Read the model definition and answer for the solid it produces. Units are mm, in the model's axes. Round coordinates to 2 decimals unless told otherwise and drop trailing zeros. Write each loop counter-clockwise with the first axis right and the second up, starting at its lowest first coordinate (ties: lowest second). Pieces come first, ordered by that corner, then holes.
from build123d import *

# Parameters (mm, degrees)
F0_R     = 1.5
F1_DEPTH = 3


with BuildPart() as f1:
    # F0 (on Top) → F1 (new body)
    with BuildSketch(Plane.XY):
        with BuildLine():
            Line((14, 6), (0, 6))
            ThreePointArc((0, 6), (-4.834596, 3.553404), (-5.726424, -1.791107))
            Line((-5.726424, -1.791107), (1.273576, -24.171107))
            ThreePointArc((1.273576, -24.171107), (7, -28.38), (12.726424, -24.171107))
            Line((12.726424, -24.171107), (19.726424, -1.791107))
            ThreePointArc((19.726424, -1.791107), (18.834596, 3.553404), (14, 6))
        make_face()
        with Locations((7, -22.38)):
            Circle(F0_R, mode=Mode.SUBTRACT)
        with Locations((7, -15)):
            Circle(F0_R, mode=Mode.SUBTRACT)
        with Locations((7, -7.62)):
            Circle(F0_R, mode=Mode.SUBTRACT)
        Circle(F0_R, mode=Mode.SUBTRACT)
        with Locations((14, 0)):
            Circle(F0_R, mode=Mode.SUBTRACT)
    extrude(amount=F1_DEPTH)


solid = f1.part
Q1. Section B-B (x = 7) is taken. Determine the outline of the cut face in (y, z), then the cut area to 3 significant figures.
Verdict:
outline: (-28.38, 0) - (-23.88, 0) - (-23.88, 3) - (-28.38, 3) - close; (-20.88, 0) - (-16.5, 0) - (-16.5, 3) - (-20.88, 3) - close; (-13.5, 0) - (-9.12, 0) - (-9.12, 3) - (-13.5, 3) - close; (-6.12, 0) - (6, 0) - (6, 3) - (-6.12, 3) - close
area: 76.1 mm2
Q2. Section D-D (y = -12) is taken. Determine the outline of the cut face in (x, z).
Verdict:
outline: (-2.53, 0) - (16.53, 0) - (16.53, 3) - (-2.53, 3) - close
Q3. Straight lines are drawn through the part: probe 1 along Y at (x, z) = (7, 0.85); probe 2 along X at (y, z) = (1, 1.95); probe 3 along X at (y, z) = (-7, 1.5). For each, find the intervals that lie inside material, in ascending order.
Verdict:
probe 1: y = -28.38 to -23.88, -20.88 to -16.5, -13.5 to -9.12, -6.12 to 6
probe 2: x = -5.92 to -1.12, 1.12 to 12.88, 15.12 to 19.92
probe 3: x = -4.1 to 5.63, 8.37 to 18.1
Q4. Section A-A (z = 1.1) is taken. Determine the outline of the cut face in (x, y), then the cut area to 3 significant figures.
Verdict:
outline: (-5.73, -1.79) - (1.27, -24.17) arc R6 ccw to (12.73, -24.17) - (19.73, -1.79) arc R6 ccw to (14, 6) - (0, 6) arc R6 ccw to start; hole circle Ø3 at (0, 0); hole circle Ø3 at (7, -22.38); hole circle Ø3 at (7, -15); hole circle Ø3 at (7, -7.62); hole circle Ø3 at (14, 0)
area: 600 mm2
Q5. Determine the mould class of faces 1 (the cylindrical face through (5.81, -8.53, 1.48)), 2 (the flat face through (7, -11, 0)), 3 (the cylindrical face through (18.88, 3.49, 1.48)) for opening direction X: pulls with the +X half, pulls with the -X half, needs draft (parallel to the pull), parting line crosses it, or undercut.
Verdict:
face 1: undercut
face 2: needs draft
face 3: pulls with the +X half
Q6. Section C-C (y = -22.38) is taken. Determine the outline of the cut face in (x, z), then the cut area to 3 significant figures.
Verdict:
outline: (0.71, 0) - (5.5, 0) - (5.5, 3) - (0.71, 3) - close; (8.5, 0) - (13.29, 0) - (13.29, 3) - (8.5, 3) - close
area: 28.7 mm2
Q7. Flat-ended cylindrical pins translate along their axes: pin 1 Ø1.5 at (y, z) = (-21, 0.5) entering from +X; pin 2 Ø1.5 at (y, z) = (-24.5, 2) entering from +X. Find the tip coordinate at first contact, or state that the pin passes through.
Verdict:
pin 1: stops at x = 13.95
pin 2: stops at x = 12.86
